Design review of the part built by this model. Coordinates are the model's own, in mm. Face numbers are marked on the shaded views. A direction names the side the tool comes from. Give positions to 0.01 mm unless a question says otherwise; leave off trailing zeros. Order: outer loops, then holes, each group sorted by start corner. A loop starts at its lowest first (then second) coordinate and runs counter-clockwise, first axis right, second up. Notation, with made-up numbers: (33.25, -2) -> (38.25, -2) arc R35 cw to (38.25, 34) -> close; hole circle Ø4 at (-31, 48.25). An arc over 180 degrees is marked (long way). Use a Markdown table: item, result. Add a question column.
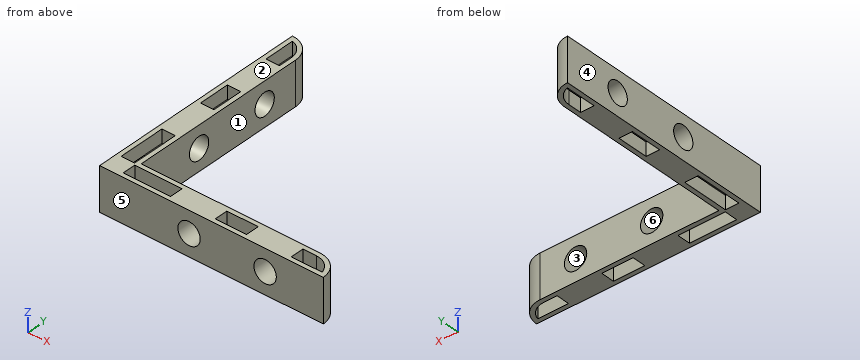
```python
from build123d import *

# Parameters (mm, degrees)
EXTRUDE_1_DEPTH        = 4.85
HOLE_WIZARD_M6_1_D     = 5
HOLE_WIZARD_M6_1_DEPTH = 23
HOLE_WIZARD_M6_1_TIP   = 1.502151548
HOLE_WIZARD_M6_2_D     = 5
HOLE_WIZARD_M6_2_DEPTH = 23
HOLE_WIZARD_M6_2_TIP   = 1.502151548
SKETCH_7_W             = 3
SKETCH_7_H             = 10.567492921
SKETCH_7_W_2           = 10.567492921
SKETCH_7_H_2           = 3
SKETCH_7_W_3           = 7
SKETCH_7_H_3           = 7
CUT_EXTRUDE_1_DEPTH    = 3
CUT_EXTRUDE_START      = -3
SKETCH_8_W             = 3
SKETCH_8_H             = 10.567492921
SKETCH_8_H_2           = 7
SKETCH_8_W_2           = 10.567492921
SKETCH_8_H_3           = 3
SKETCH_8_W_3           = 7
CUT_EXTRUDE_2_DEPTH    = 3


with BuildPart() as part:
    # 草图1 → 凸台-拉伸1 (new, symmetric)
    with BuildSketch(Plane.XY):
        with BuildLine():
            Line((0, 50), (0, 0))
            Line((0, 0), (50, 0))
            ThreePointArc((50, 0), (48.535533906, 3.535533906), (45, 5))
            Line((45, 5), (5, 5))
            Line((5, 5), (5, 45))
            ThreePointArc((5, 45), (3.535533906, 48.535533906), (0, 50))
        make_face()
    extrude(amount=EXTRUDE_1_DEPTH, both=True)

    # M6 螺纹孔1
    with Locations(Plane(origin=(5, 37, 0), x_dir=(0, 0, 1), z_dir=(1, 0, 0))):
        with Locations((0, 0), (0, 17)):
            Hole(HOLE_WIZARD_M6_1_D / 2, depth=HOLE_WIZARD_M6_1_DEPTH)
            with Locations((0, 0, -(HOLE_WIZARD_M6_1_DEPTH + HOLE_WIZARD_M6_1_TIP / 2))):  # 118° drill point
                Cone(0, HOLE_WIZARD_M6_1_D / 2, HOLE_WIZARD_M6_1_TIP, mode=Mode.SUBTRACT)

    # M6 螺纹孔2
    with Locations(Plane(origin=(20, 5, 0), x_dir=(0, 0, 1), z_dir=(0, 1, 0))):
        with Locations((0, 0), (0, 17)):
            Hole(HOLE_WIZARD_M6_2_D / 2, depth=HOLE_WIZARD_M6_2_DEPTH)
            with Locations((0, 0, -(HOLE_WIZARD_M6_2_DEPTH + HOLE_WIZARD_M6_2_TIP / 2))):  # 118° drill point
                Cone(0, HOLE_WIZARD_M6_2_D / 2, HOLE_WIZARD_M6_2_TIP, mode=Mode.SUBTRACT)

    # 草图7 → 切除-拉伸1 (cut)
    with BuildSketch(Plane(origin=(0, 0, -4.85), x_dir=(-1, 0, 0), z_dir=(0, 0, -1))):
        with Locations((-2.5, 9.71625354)):
            Rectangle(SKETCH_7_W, SKETCH_7_H)
        with Locations((-9.71625354, 2.5)):
            Rectangle(SKETCH_7_W_2, SKETCH_7_H_2)
        with BuildLine():
            Line((-4, 42), (-1, 42))
            Line((-1, 42), (-1, 48.872983346))
            ThreePointArc((-1, 48.872983346), (-3.16227766, 47.449489743), (-4, 45))
            Line((-4, 45), (-4, 42))
        make_face()
        with BuildLine():
            Line((-42, 4), (-42, 1))
            Line((-42, 1), (-48.872983346, 1))
            ThreePointArc((-48.872983346, 1), (-47.449489743, 3.16227766), (-45, 4))
            Line((-45, 4), (-42, 4))
        make_face()
        with Locations((-28.5, 2.5)):
            Rectangle(SKETCH_7_W_3, SKETCH_7_H_2)
        with Locations((-2.5, 28.5)):
            Rectangle(SKETCH_7_W, SKETCH_7_H_3)
    extrude(amount=-CUT_EXTRUDE_1_DEPTH, mode=Mode.SUBTRACT)

    # 草图8 → 切除-拉伸2 (cut)
    with BuildSketch(Plane.XY.offset(4.85).offset(CUT_EXTRUDE_START)):
        with BuildLine():
            Line((1, 42), (1, 48.872983346))
            ThreePointArc((1, 48.872983346), (3.16227766, 47.449489743), (4, 45))
            Line((4, 45), (4, 42))
            Line((4, 42), (1, 42))
        make_face()
        with BuildLine():
            Line((42, 4), (45, 4))
            ThreePointArc((45, 4), (47.449489743, 3.16227766), (48.872983346, 1))
            Line((48.872983346, 1), (42, 1))
            Line((42, 1), (42, 4))
        make_face()
        with Locations((2.5, 9.71625354)):
            Rectangle(SKETCH_8_W, SKETCH_8_H)
        with Locations((2.5, 28.5)):
            Rectangle(SKETCH_8_W, SKETCH_8_H_2)
        with Locations((9.71625354, 2.5)):
            Rectangle(SKETCH_8_W_2, SKETCH_8_H_3)
        with Locations((28.5, 2.5)):
            Rectangle(SKETCH_8_W_3, SKETCH_8_H_3)
    extrude(amount=CUT_EXTRUDE_2_DEPTH, mode=Mode.SUBTRACT)


solid = part.part
```
1) The part is to be moulded in two halves that separate along X. For the marked faces 3, 4, 5 and 6, say which applies: +X half, -X half, draft (parallel to the pull), parting line (faces both ways), or undercut.
2) Add section C-C (z = 0). Give the boundary of the cut face in (x, y), then the cut area to 3 significant figures.
3) Add section D-D (x = 12). Give the boundary of the cut face in (y, z).
4) For L1, parallel to X at y = 11, z = 2.5; L2, parallel to Y at x = 3.5, z = -4.25, list the stretches that pass through material, from the lowest coordinate up. Write a range as [from, to].
5) Insertion check: pin 1 (3.5 mm diameter, centred on x = 2.5, z = 3, fed in from -Y); pin 2 (0.9 mm diameter, centred on y = 2, z = -4, fed in from +X); pin 3 (2 mm diameter, centred on y = 18, z = 3, fed in from +X); pin 4 (5 mm diameter, centred on x = 27.5, z = -3, fed in from +Y). Each pin has a flat end and moves straight along its axis. Give the tip position at first contact, or say it passes through.
6) Machinability: for the marked faces 1 and 2, which of the approach directions +Z, -Z, +X, -X, +Y, -Y give a long, thin tool a straight path to every point of the face, cutting with its end or side? Answer none if there is none.
7) Add section A-A (y = 20). Give the boundary of the cut face in (x, z).
Worked answers:
| question | item | result |
|---|---|---|
| 1 | face 3 | undercut |
| 1 | face 4 | -X half |
| 1 | face 5 | draft |
| 1 | face 6 | undercut |
| 2 | outline | (0, 0) -> (17.5, 0) -> (17.5, 5) -> (5, 5) -> (5, 17.5) -> (0, 17.5) -> close; (0, 22.5) -> (5, 22.5) -> (5, 34.5) -> (0, 34.5) -> close; (0, 39.5) -> (5, 39.5) -> (5, 45) arc R5 ccw to (0, 50) -> close; (22.5, 0) -> (34.5, 0) -> (34.5, 5) -> (22.5, 5) -> close; (39.5, 0) -> (50, 0) arc R5 ccw to (45, 5) -> (39.5, 5) -> close |
| 2 | area | 364 mm^2 |
| 3 | outline | (0, -4.85) -> (1, -4.85) -> (1, -1.85) -> (4, -1.85) -> (4, -4.85) -> (5, -4.85) -> (5, 4.85) -> (4, 4.85) -> (4, 1.85) -> (1, 1.85) -> (1, 4.85) -> (0, 4.85) -> close |
| 4 | L1 | [0, 1], [4, 5] |
| 4 | L2 | [0, 4.43], [15, 25], [32, 42], [46.94, 48.57] |
| 5 | pin 1 | y = 0 |
| 5 | pin 2 | x = 49.75 |
| 5 | pin 3 | x = 5 |
| 5 | pin 4 | y = 5 |
| 6 | face 1 | +Z, -Z, +X, +Y |
| 6 | face 2 | +Z, +X, -X, +Y, -Y |
| 7 | outline | (0, -4.85) -> (5, -4.85) -> (5, -2.5) -> (0, -2.5) -> close; (0, 2.5) -> (5, 2.5) -> (5, 4.85) -> (0, 4.85) -> close |
